Autodesk Inventor part; units mm, degrees
ref_plane "YZ Plane" through (0, 0, 0) normal (1, 0, 0) x (0, 1, 0)
ref_plane "XZ Plane" through (0, 0, 0) normal (0, 1, 0) x (-1, 0, 0)
ref_plane "XY Plane" through (0, 0, 0) normal (0, 0, 1) x (1, 0, 0)
sketch "Sketch1" plane through (0, 0, 0) normal (0, 0, 1) x (1, 0, 0)
  line L0 (0, 0) -> (-390, 0)
  line L1 (0, -80) -> (0, 0)
  line L2 (-390, 0) -> (-390, -80)
  line L3 (-390, -80) -> (0, -80)
  point P0 (0, -40)
  dimension "d32" = 80
  dimension "d60" = 80
  dimension "d61" = 390
extrude "Plate1" add sketch "Sketch1" along normal blind 2
sketch "Sketch8" plane through (0, 0, 2) normal (0, 0, 1) x (1, 0, 0)
  line L0 (-79.75, -48.25) -> (-110.25, -48.25)
  line L1 (-110.25, -48.25) -> (-110.25, -17.75)
  line L2 (-110.25, -17.75) -> (-79.75, -17.75)
  line L3 (-79.75, -17.75) -> (-79.75, -48.25)
  line L4 (-79.75, -48.25) -> (-110.25, -17.75) construction
  line L5 (-110.25, -48.25) -> (-79.75, -17.75) construction
  circle A0 centre (-72, -56) radius 2.5
  circle A1 centre (-118, -56) radius 2.5
  circle A2 centre (-118, -10) radius 2.5
  circle A3 centre (-72, -10) radius 2.5
  line L6 (0, 0) -> (0, -80)
  line L7 (-390, 0) -> (0, 0)
  line L8 (-110.25, -48.25) -> (-118, -56) construction
  line L9 (-118, -10) -> (-72, -10) construction
  line L10 (-72, -10) -> (-72, -56) construction
  line L11 (-72, -56) -> (-118, -56) construction
  line L12 (-118, -56) -> (-118, -10) construction
  point P0 (-95, -33)
  dimension "d51" = 30.5
  dimension "d52" = 30.5
  dimension "d53" = 5
  dimension "d72" = 95
  dimension "d78" = 46
  dimension "d79" = 10
extrude "Cut3" cut sketch "Sketch8" against normal blind 2
pattern_linear "Rectangular Pattern1" count 3 spacing 120 along (-1, 0, 0) of "Cut3"
sketch "Sketch9" plane through (0, -2, 2) normal (0, 1, 0) x (-1, 0, 0)
  line L0 (390, 0) -> (0, 0)
  line L1 (0, 0) -> (0, -75)
  line L2 (0, -75) -> (390, -75)
  line L3 (390, -75) -> (390, 0)
edge flange "Flange3" height 75 angle 90 thickness 2 bend radius 2.75 thickness toward (0, 1, 0) relief round relief width 2 relief depth 1 edges at (-195, 0, 0) wall of the first edge with corners at (-390, -2, 2) (0, -2, 2) (0, -2, -73) (-390, -2, -73)
bend "Bend3"
corner "Corner3"
equation "\"d51\" = d52"
equation "\"d55\" = Thickness"
equation "\"d2\" = Thickness"
equation "\"d62\" = BendReliefWidth"
equation "\"d63\" = BendReliefDepth"
equation "\"d64\" = MinimumRemnant"
equation "\"d65\" = TransitionRadius"
equation "\"d68\" = BendRadius"
equation "\"d69\" = CornerReliefSize"
equation "\"d70\" = GapSize"
equation "\"d71\" = JacobiRadiusSize"
equation "\"BendReliefWidth\" = Thickness"
equation "\"BendReliefDepth\" = 0.5 * Thickness"
equation "\"CornerReliefSize\" = 4 * Thickness"
equation "\"MinimumRemnant\" = 2 * Thickness"
equation "\"TransitionRadius\" = BendRadius"
equation "\"JacobiRadiusSize\" = BendRadius"
equation "\"GapSize\" = Thickness"
properties part number "PRS-1422 BOTTOM FDS diameter way up_CPY" material "Stainless Steel"
Input: part model. Units: mm. Frame: model coordinates. A direction names the side the tool comes from. Give positions to 0.01 mm unless a question says otherwise; leave off trailing zeros. Order: outer loops, then holes, each group sorted by start corner. A loop starts at its lowest first (then second) coordinate and runs counter-clockwise, first axis right, second up. Notation, with made-up numbers: M -7.5,37.25 L 40.5,37.25 A21 cw 40.5,42.25 Z; hole C 32,79.25 d7. An arc over 180 degrees is marked long. Answer as a JSON object with one key per item and string values.
1. First-contact query: P1, Ø2, axis at x = -218.5, y = -47, coming from the +Z side; P2, Ø2, axis at x = -283, z = -61.5, coming from the -Y side; P3, Ø6, axis at x = -72, y = -10, coming from the -Z side. Flat tips, straight axial feed; report the tip coordinate or a pass-through.
Result sheet:
{"P1": "through", "P2": "y = -2", "P3": "z = 0"}
2. Ray query, line 1 (Y direction, x = -358, z = 0.8); line 2 (Y direction, x = -72, z = 1); line 3 (Y direction, x = -310, z = -9). Return the intervals inside material, ascending. Write a range as [from, to].
Result sheet:
{"line 1": "[-80, -58.5], [-53.5, -12.5], [-7.5, -1.59]", "line 2": "[-80, -58.5], [-53.5, -12.5], [-7.5, -1.83]", "line 3": "[-2, 0]"}
3. Reachability of faces 1 (the flat face through (-198, -42, 0)), 2 (the flat face through (0, -22, 0.4)) from +Z, -Z, +X, -X, +Y, -Y: full face, straight path, thin tool, end or side. Return the list, or none.
Result sheet:
{"face 1": "-Z, +X, -X, -Y", "face 2": "+Z, -Z, +X, +Y, -Y"}
4. Cut plane A-A, the plane x = -327. Output: boundary loops of the cut face in (y, z).
Result sheet:
{"outline": "M -80,0 L -48.25,0 L -48.25,2 L -80,2 Z; M -17.75,0 L -4.75,0 A2.75 cw -2,-2.75 L -2,-73 L 0,-73 L 0,-2.75 A4.75 ccw -4.75,2 L -17.75,2 Z"}
5. Cut plane B-B, the plane z = -30. Output: boundary loops of the cut face in (x, y), and give its area (3 significant figures).
Result sheet:
{"outline": "M -390,-2 L 0,-2 L 0,0 L -390,0 Z", "area": "780 mm²"}
